Design review of the part built by this model. Coordinates are the model's own, in mm. A direction names the side the tool comes from. Give positions to 0.01 mm unless a question says otherwise; leave off trailing zeros. Order: outer loops, then holes, each group sorted by start corner. A loop starts at its lowest first (then second) coordinate and runs counter-clockwise, first axis right, second up.
```python
from build123d import *

# Parameters (mm, degrees)
F0_R         = 55
F1_DEPTH     = 6
F2_R         = 5
F3_DEPTH     = 6
F5_DEPTH     = 8
F7_R         = 55
F7_R_2       = 54.4
F8_DEPTH     = 4
F10_DEPTH    = 25
F11_R        = 5
F12_T1_DEPTH = 6
F13_R        = 2


# Not quite as in the source:
# - a fillet or chamfer that OpenCascade refuses, or shapes differently, is made with other operations: its cross-section is extruded or revolved along the edge and cut away or added


with BuildPart() as f1:
    # F0 (on Top) → F1 (new body)
    with BuildSketch(Plane.XY):
        Circle(F0_R)
    extrude(amount=F1_DEPTH)

    # F2 (on face) → F3 (join)
    with BuildSketch(Plane.XY.offset(6)):
        Circle(F2_R)
    extrude(amount=F3_DEPTH)

    # F4 (on face) → F5 (cut)
    with BuildSketch(Plane.XY.offset(12)):
        with BuildLine():
            Line((2.1498313887, 1.825), (-2.1498313887, 1.825))
            ThreePointArc((-2.1498313887, 1.825), (-2.82, 0), (-2.1498313887, -1.825))
            Line((-2.1498313887, -1.825), (2.1498313887, -1.825))
            ThreePointArc((2.1498313887, -1.825), (2.82, 0), (2.1498313887, 1.825))
        make_face()
    extrude(amount=-F5_DEPTH, mode=Mode.SUBTRACT)

    # F7 (on offset) → F8 (cut)
    with BuildSketch(Plane.XY.offset(1)):
        Circle(F7_R)
        Circle(F7_R_2, mode=Mode.SUBTRACT)
    extrude(amount=F8_DEPTH, mode=Mode.SUBTRACT)

    # F9 (on face) → F10 (cut)
    with BuildSketch(Plane.XY.offset(6)):
        with BuildLine():
            Line((7.1352549156, 7.0062926922), (41.9971112805, 27.1337948489))
            ThreePointArc((41.9971112805, 27.1337948489), (0, 50.0000017881), (-41.9971112805, 27.1337948489))
            Line((-41.9971112805, 27.1337948489), (-7.1352549156, 7.0062926922))
            ThreePointArc((-7.1352549156, 7.0062926922), (0, 10), (7.1352549156, 7.0062926922))
        make_face()
        with BuildLine():
            ThreePointArc((2.5, -49.937462679), (36.2284431303, -34.460123145), (50.0000017881, 0))
            ThreePointArc((50.0000017881, 0), (48.6048136629, 11.729120496), (44.4971112805, 22.80366783))
            Line((44.4971112805, 22.80366783), (9.6352549156, 2.6761656733))
            ThreePointArc((9.6352549156, 2.6761656733), (9.9083941473, 1.3504537837), (10, 0))
            ThreePointArc((10, 0), (7.9056941504, -6.123724357), (2.5, -9.6824583655))
            Line((2.5, -9.6824583655), (2.5, -49.937462679))
        make_face()
        with BuildLine():
            ThreePointArc((-44.4971112805, 22.80366783), (-43.3012717378, -25.0000008941), (-2.5, -49.937462679))
            Line((-2.5, -49.937462679), (-2.5, -9.6824583655))
            ThreePointArc((-2.5, -9.6824583655), (-8.6602540378, -5), (-9.6352549156, 2.6761656733))
            Line((-9.6352549156, 2.6761656733), (-44.4971112805, 22.80366783))
        make_face()
    extrude(amount=-F10_DEPTH, mode=Mode.SUBTRACT)

    # F11
    f11_edges = [f1.edges().sort_by_distance(p)[0] for p in [
        (-44.497111, 22.803668, 3),
        (-41.997111, 27.133795, 3),
        (41.997111, 27.133795, 3),
        (44.497111, 22.803668, 3),
        (2.5, -49.937463, 3),
        (-2.5, -49.937463, 3),
    ]]
    fillet(f11_edges, radius=F11_R)

    # F12: fillet of radius 5 on 6 edges, made by hand

    # F12_s2 → F12_t1 (join)
    with BuildSketch(Plane.XY):
        with BuildLine():
            ThreePointArc((-12.5, 4.3301270189), (-10.6698729811, 2.5), (-10, 0))
            ThreePointArc((-10, 0), (-9.9083941473, 1.3504537837), (-9.6352549156, 2.6761656733))
            Line((-9.6352549156, 2.6761656733), (-12.5, 4.3301270189))
        make_face()
        with BuildLine():
            ThreePointArc((-5, -8.6602540378), (-3.1698729811, -10.4903810568), (-2.5, -12.9903810568))
            Line((-2.5, -12.9903810568), (-2.5, -9.6824583655))
            ThreePointArc((-2.5, -9.6824583655), (-3.7846697903, -9.2561479341), (-5, -8.6602540378))
        make_face()
        with BuildLine():
            ThreePointArc((2.5, -12.9903810568), (3.1698729811, -10.4903810568), (5, -8.6602540378))
            ThreePointArc((5, -8.6602540378), (3.7846697903, -9.2561479341), (2.5, -9.6824583655))
            Line((2.5, -9.6824583655), (2.5, -12.9903810568))
        make_face()
        with BuildLine():
            ThreePointArc((12.5, 4.3301270189), (10.6698729811, 2.5), (10, 0))
            ThreePointArc((10, 0), (9.9083941473, 1.3504537837), (9.6352549156, 2.6761656733))
            Line((9.6352549156, 2.6761656733), (12.5, 4.3301270189))
        make_face()
        with BuildLine():
            ThreePointArc((10, 8.6602540378), (7.5, 7.9903810568), (5, 8.6602540378))
            ThreePointArc((5, 8.6602540378), (6.123724357, 7.9056941504), (7.1352549156, 7.0062926922))
            Line((7.1352549156, 7.0062926922), (10, 8.6602540378))
        make_face()
        with BuildLine():
            ThreePointArc((-10, 8.6602540378), (-7.5, 7.9903810568), (-5, 8.6602540378))
            ThreePointArc((-5, 8.6602540378), (-6.123724357, 7.9056941504), (-7.1352549156, 7.0062926922))
            Line((-7.1352549156, 7.0062926922), (-10, 8.6602540378))
        make_face()
    extrude(amount=F12_T1_DEPTH)

    # F13
    f13_edges = [f1.edges().sort_by_distance(p)[0] for p in [
        (-5, 0, 6),
        (-5, 0, 12),
    ]]
    fillet(f13_edges, radius=F13_R)


solid = f1.part
```
1. Take a section at B-B (y = -32). State the section outline as (x, z) points, then the cut area to 3 significant figures.
Recorded:
outline: (-44.73, 0) - (-38.42, 0) - (-38.42, 6) - (-44.73, 6) - (-44.73, 5) - (-43.99, 5) - (-43.99, 1) - (-44.73, 1) - close; (-2.5, 0) - (2.5, 0) - (2.5, 6) - (-2.5, 6) - close; (38.42, 0) - (44.73, 0) - (44.73, 1) - (43.99, 1) - (43.99, 5) - (44.73, 5) - (44.73, 6) - (38.42, 6) - close
area: 99.8 mm2
2. Draft analysis for pull direction Z (two halves, no side actions). For faces 1 (the face through (-53.2, 12.5, 5)), 2 (the face through (0, 0, 4)), 3 (the face through (-11.793, -53.106, 2.972)), 4 (the face through (-4.32, -48.23, 2.96)), state which applies: pulls with the +Z half, pulls with the -Z half, needs draft (parallel to the pull), parting line crosses it, or undercut.
Recorded:
face 1: undercut
face 2: pulls with the +Z half
face 3: undercut
face 4: needs draft
3. For line 1 along X through (y, z) = (11, 3.25) (3 decimals); line 2 along X through (y, z) = (7.5, 3); line 3 along X through (y, z) = (-39.5, 4), list the stretches that pass through material, from the lowest coordinate up.
Recorded:
line 1: x = -53.276 to -48.775, -24.053 to -14.053, 14.053 to 24.053, 48.775 to 53.276
line 2: x = -53.88 to -49.43, -17.99 to 17.99, 49.43 to 53.88
line 3: x = -37.4 to -30.66, -2.5 to 2.5, 30.66 to 37.4
4. For pin 1 (3 mm diameter, centred on y = -32, z = 3, fed in from -X); pin 2 (1 mm diameter, centred on x = -1, z = 10.5, fed in from -Y); pin 3 (1 mm diameter, centred on x = -13, z = 8, fed in from +Y); pin 4 (2 mm diameter, centred on y = 2, z = 3.5, fed in from -X), all flat-tipped, find the tip position at first contact; note any pin that passes through.
Recorded:
pin 1: stops at x = -45.05
pin 2: stops at y = -4.95
pin 3: passes through
pin 4: stops at x = -54.39
5. Machinability: for faces 5 (the face through (0, -1.825, 8)), 6 (the face through (43.927, 20.374, 2.958)), 7 (the face through (0, -4, 0)), which of the approach directions +Z, -Z, +X, -X, +Y, -Y give a long, thin tool a straight path to every point of the face, cutting with its end or side? Answer none if there is none.
Recorded:
face 5: +Z
face 6: +Z, -Z
face 7: -Z, +X, -X, +Y, -Y
6. Take a section at C-C (x = -21.5). State the section outline as (y, z) points.
Recorded:
outline: (-50.62, 0) - (-45.14, 0) - (-45.14, 6) - (-50.62, 6) - (-50.62, 5) - (-49.97, 5) - (-49.97, 1) - (-50.62, 1) - close; (9.53, 0) - (15.3, 0) - (15.3, 6) - (9.53, 6) - close; (45.14, 0) - (50.62, 0) - (50.62, 1) - (49.97, 1) - (49.97, 5) - (50.62, 5) - (50.62, 6) - (45.14, 6) - close
7. Take a section at A-A (x = 0). State the section outline as (y, z) points (3 decimals).
Recorded:
outline: (-55, 0) - (10, 0) - (10, 6) - (7, 6) arc R2 cw to (5, 8) - (5, 10) arc R2 ccw to (3, 12) - (1.825, 12) - (1.825, 4) - (-1.825, 4) - (-1.825, 12) - (-3, 12) arc R2 ccw to (-5, 10) - (-5, 8) arc R2 cw to (-7, 6) - (-55, 6) - (-55, 5) - (-54.4, 5) - (-54.4, 1) - (-55, 1) - close; (50, 0) - (55, 0) - (55, 1) - (54.4, 1) - (54.4, 5) - (55, 5) - (55, 6) - (50, 6) - close
